Autodesk Inventor part; units mm, degrees
ref_plane "Work Plane1" through (0, 0, 10.47) normal (0, 0, 1) x (1, 0, 0)
ref_plane "YZ Plane" through (0, 0, 0) normal (1, 0, 0) x (0, 1, 0)
ref_plane "XZ Plane" through (0, 0, 0) normal (0, 1, 0) x (-1, 0, 0)
sketch "Base" plane through (0, 0, 0) normal (0, 0, 1) x (1, 0, 0)
  line L0 (-26.9, -20.25) -> (26.9, -20.25)
  line L1 (26.9, -20.25) -> (26.9, 20.25)
  line L2 (26.9, 20.25) -> (-26.9, 20.25)
  line L3 (-26.9, 20.25) -> (-26.9, -20.25)
  line L4 (-26.9, -20.25) -> (26.9, 20.25) construction
  line L5 (26.9, -20.25) -> (-26.9, 20.25) construction
  line L6 (-25.4, 16.25) -> (-22.9, 16.25) construction
  line L7 (-22.9, 16.25) -> (-22.9, 18.75) construction
  line L8 (-22.9, 18.75) -> (-25.4, 18.75) construction
  line L9 (-25.4, 18.75) -> (-25.4, 16.25) construction
  line L10 (-25.4, 16.25) -> (-22.9, 18.75) construction
  line L11 (-22.9, 16.25) -> (-25.4, 18.75) construction
  circle A0 centre (-24.15, 17.5) radius 1.25
  line L12 (-26.9, 0) -> (0, 0) construction
  line L13 (0, 20.25) -> (0, 0) construction
  circle A1 centre (-24.15, -17.5) radius 1.25
  circle A2 centre (24.15, 17.5) radius 1.25
  circle A3 centre (24.15, -17.5) radius 1.25
  point P0 (-25.4, 17.5)
  dimension "d0" = 53.8
  dimension "d1" = 40.5
  dimension "d2" = 1.5
  dimension "d3" = 1.5
  dimension "d4" = 2.5
extrude "BaseFeature" add sketch "Base" along normal blind 1.67
fillet "Fillet1" radius 2.5 4 edges at (-26.9, -20.25, 0.835) (26.9, -20.25, 0.835) (-26.9, 20.25, 0.835) (26.9, 20.25, 0.835)
sketch "Sketch2" plane through (0, 0, 1.67) normal (0, 0, 1) x (1, 0, 0)
  line L0 (-26.9, 17.75) -> (-26.9, -17.75)
  line L1 (-26.9, 0) -> (0, 0) construction
  line L2 (-26.4, 8.05) -> (-19.6, 8.05)
  line L3 (-19.6, 8.05) -> (-19.6, 1.25)
  line L4 (-19.6, 1.25) -> (-26.4, 1.25)
  line L5 (-26.4, 1.25) -> (-26.4, 8.05)
  line L6 (-26.4, -8.05) -> (-19.6, -8.05)
  line L7 (-19.6, -8.05) -> (-19.6, -1.25)
  line L8 (-19.6, -1.25) -> (-26.4, -1.25)
  line L9 (-26.4, -1.25) -> (-26.4, -8.05)
  dimension "d8" = 1.25
  dimension "d9" = 0.5
  dimension "d10" = 6.8
extrude "Extrusion2" add sketch "Sketch2" along normal blind 4.8
ref_plane "Work Plane1" through (0, 0, 10.47) normal (0, 0, 1) x (1, 0, 0)
sketch "Sketch3" plane through (0, 0, 10.47) normal (0, 0, 1) x (1, 0, 0)
  line L0 (-26.4, 8.05) -> (-19.6, 8.05)
  line L1 (-23, 8.05) -> (-23, 1.25) construction
  line L2 (-19.6, 1.25) -> (-26.4, 1.25)
  line L3 (-37.66, 0) -> (37.66, 0) construction
  line L4 (-26.4, 1.25) -> (-19.6, 1.25)
  line L5 (-19.6, 1.25) -> (-19.6, 8.05)
  line L6 (-19.6, 8.05) -> (-26.4, 8.05)
  line L7 (-26.4, 8.05) -> (-26.4, 1.25)
  line L8 (-25, 8.05) -> (-21, 8.05)
  line L9 (-21, 8.05) -> (-21, 1.25)
  line L10 (-21, 1.25) -> (-25, 1.25)
  line L11 (-25, 1.25) -> (-25, 8.05)
  point P0 (0, 0)
  dimension "d14" = 4
sketch "Sketch4" plane through (0, 0, 6.47) normal (0, 0, 1) x (1, 0, 0)
  line L0 (-26.4, 1.25) -> (-19.6, 1.25)
  line L1 (-19.6, 1.25) -> (-19.6, 8.05)
  line L2 (-19.6, 8.05) -> (-26.4, 8.05)
  line L3 (-26.4, 8.05) -> (-26.4, 1.25)
  point P0 (0, 0)
loft "Loft1" add profiles "Sketch3" section 2 edges at (-23, 1.25, 6.47) (-19.6, 4.65, 6.47) (-23, 8.05, 6.47) (-26.4, 4.65, 6.47) contours L0 L9 L2 L11
mirror "Mirror1" about plane through (0, 0, 0) normal (0, 1, 0) of "Loft1"
sketch "Sketch5" plane through (-25, 1.25, 10.47) normal (0, 0, 1) x (1, 0, 0)
  line L0 (0, 6.8) -> (0, 0)
  line L1 (0, 0) -> (4, 0)
  line L2 (4, 0) -> (4, 6.8)
  line L3 (4, 6.8) -> (0, 6.8)
  line L4 (-12.66, -1.25) -> (62.66, -1.25) construction
  line L5 (2, 6.8) -> (2, 0) construction
  circle A0 centre (2, 5.025) radius 1.5
  line L6 (0, 3.4) -> (4, 3.4) construction
  circle A1 centre (2, 1.775) radius 1.5
  point P0 (25, -1.25)
  dimension "d19" = 3
  dimension "d20" = 3.25
extrude "Extrusion3" cut sketch "Sketch5" against normal blind 3 contours A0 | A1
mirror "Mirror2" about plane through (0, 0, 0) normal (0, 1, 0) of "Extrusion3"
sketch "Sketch6" plane through (0, 0, 1.67) normal (0, 0, 1) x (1, 0, 0)
  line L0 (-24.4, -20.25) -> (24.4, -20.25)
  line L1 (-26.9, 17.75) -> (-26.9, -17.75)
  circle A0 centre (-14.4, -16.15) radius 4
  line L2 (-18.4, -16.15) -> (-18.4, -20.25) construction
  point P0 (0, 0)
  dimension "d23" = 8
  dimension "d24" = 4.1
  dimension "d25" = 8.5
extrude "Extrusion4" add sketch "Sketch6" along normal blind 12
fillet "Fillet2" radius 0.5 1 edges at (-18.4, -16.15, 13.67)
sketch "Sketch7" plane through (0, 0, 1.67) normal (0, 0, 1) x (1, 0, 0)
  line L0 (7.2, -9.65) -> (16.2, -9.65)
  line L1 (16.2, -9.65) -> (16.2, -23.65)
  line L2 (16.2, -23.65) -> (7.2, -23.65)
  line L3 (7.2, -23.65) -> (7.2, -9.65)
  line L4 (7.2, -23.65) -> (16.2, -23.65)
  line L5 (16.2, -23.65) -> (16.2, -20.25)
  line L6 (16.2, -20.25) -> (7.2, -20.25)
  line L7 (7.2, -20.25) -> (7.2, -23.65)
  line L8 (-24.4, -20.25) -> (24.4, -20.25)
  line L9 (26.9, -17.75) -> (26.9, 17.75)
  point P0 (0, 0)
  point P1 (11.7, -23.65)
  dimension "d29" = 9
  dimension "d30" = 14
  dimension "d31" = 3.4
  dimension "d32" = 10.7
extrude "Extrusion5" add sketch "Sketch7" along normal blind 10.7
sketch "Sketch8" plane through (7.2, -23.65, 1.67) normal (0, -1, 0) x (1, 0, 0)
  line L0 (0, 0) -> (9, 0)
  line L1 (9, 0) -> (9, 10.7)
  line L2 (0, 10.7) -> (9, 10.7)
  line L3 (0, 0) -> (0, 10.7)
  line L4 (4.5, 10.7) -> (4.5, 0) construction
  circle A0 centre (4.5, 6.2) radius 3.85
  point P0 (-7.2, -1.67)
  dimension "d35" = 7.7
  dimension "d36" = 4.5
extrude "Extrusion6" cut sketch "Sketch8" against normal blind 10.7 contours A0
sketch "Sketch9" plane through (0, 0, 1.67) normal (0, 0, 1) x (1, 0, 0)
  line L0 (11.77, 7.05) -> (29.4, 7.05)
  line L1 (29.4, 7.05) -> (29.4, 13.37)
  line L2 (29.4, 13.37) -> (11.77, 13.37)
  line L3 (11.77, 13.37) -> (11.77, 7.05)
  line L4 (24.4, 20.25) -> (-24.4, 20.25)
  line L5 (26.9, 13.37) -> (26.9, 7.05)
  line L6 (26.9, -17.75) -> (26.9, 17.75)
  point P0 (0, 0)
  dimension "d39" = 13.2
  dimension "d40" = 6.32
  dimension "d41" = 17.63
  dimension "d42" = 2.5
extrude "Extrusion7" add sketch "Sketch9" along normal blind 5 contours L3 L2 L5 L0
sketch "Sketch10" plane through (26.9, -17.75, 0) normal (1, 0, 0) x (0, 0, -1)
  line L0 (-1.67, 24.8) -> (-6.67, 24.8) construction
  line L1 (-1.67, 31.12) -> (-6.67, 31.12) construction
  line L2 (-6.67, 24.8) -> (-1.67, 31.12) construction
  circle A0 centre (-4.17, 27.96) radius 1.8
  point P0 (0, 17.75)
  dimension "d45" = 3.6
extrude "Extrusion8" cut sketch "Sketch10" against normal blind 5
sketch "Sketch11" plane through (26.9, -17.75, 0) normal (1, 0, 0) x (0, 0, -1)
  circle A0 centre (-4.17, 27.96) radius 1.8
  line L0 (-6.67, 24.8) -> (-6.67, 31.12)
  circle A1 centre (-4.17, 27.96) radius 2.5
  point P0 (0, 17.75)
extrude "Extrusion9" add sketch "Sketch11" along normal blind 2.5
sketch "Sketch12" plane through (0, 0, 0) normal (0, 0, -1) x (-1, 0, 0)
  line L0 (-26.9, 13.75) -> (-17.4, 13.75)
  line L1 (-17.4, 13.75) -> (-17.4, 4.25)
  line L2 (-17.4, 4.25) -> (-26.9, 4.25)
  line L3 (-26.9, 4.25) -> (-26.9, 13.75)
  line L4 (-26.9, -17.75) -> (-26.9, 17.75)
  line L5 (-24.4, 20.25) -> (24.4, 20.25)
  point P0 (0, 0)
  dimension "d50" = 9.5
  dimension "d51" = 6.5
extrude "Extrusion10" add sketch "Sketch12" along normal blind 5
sketch "Sketch13" plane through (0, 0, -5) normal (0, 0, -1) x (-1, 0, 0)
  line L0 (-17.4, 13.75) -> (-26.9, 13.75)
  line L1 (-26.9, 13.75) -> (-26.9, 4.25)
  line L2 (-26.9, 4.25) -> (-17.4, 4.25)
  line L3 (-17.4, 4.25) -> (-17.4, 13.75)
  circle A0 centre (-22.15, 9) radius 4
  line L4 (-17.4, 13.75) -> (-17.4, 4.25)
  line L5 (-26.9, 13.75) -> (-17.4, 4.25) construction
  point P0 (0, 0)
  dimension "d54" = 8
extrude "Extrusion11" add sketch "Sketch13" along normal blind 5 draft -4 contours A0
properties part number "FaceAudioBoard"
Here's how the part is built. I have some questions about the finished solid (model axes, mm). A direction names the side the tool comes from. Coordinates: 2 decimals unless noted, no trailing zeros. Order: outer loops, then holes, each group sorted by start corner. A loop starts at its lowest first (then second) coordinate and runs counter-clockwise, first axis right, second up. Notation, with made-up numbers: (71.25, -32.5) -> (78.25, -32.5) arc R21 cw to (78.25, -0.5) -> close; hole circle Ø6 at (-27.5, 21.5). An arc over 180 degrees is marked (long way). Return JSON: item names as keys, results as strings.
1) Thinking about a two-plate mould opening in X: for faces 5 (the cylindrical face through (26.187, 19.498, 0.847)), 6 (the flat face through (19, 13.37, 4)), 7 (the flat face through (7.2, -17, 7)), which applies, +X half, -X half, draft (parallel to the pull), parting line (faces both ways), or undercut?
Conclusion:
{"face 5": "+X half", "face 6": "draft", "face 7": "undercut"}
2) I'm going to push flat-ended pins straight in: P1, Ø1, axis at x = 19, z = 0, coming from the -Y side; P2, Ø5.5, axis at x = 24.5, z = -3.5, coming from the +Y side; P3, Ø6, axis at x = -9, y = 12, coming from the +Z side. Where does each tip first touch, or does it pass through?
Conclusion:
{"P1": "stops at y = -20.25", "P2": "stops at y = 13.75", "P3": "stops at z = 1.67"}
3) If we section it at A-A on z = 9.25: List the corners of the cut face in (x, y) for me (3 decimals).
Conclusion:
{"outline": "(-25.427, -8.05) -> (-20.573, -8.05) -> (-20.573, -1.25) -> (-25.427, -1.25) -> close; (-25.427, 1.25) -> (-20.573, 1.25) -> (-20.573, 8.05) -> (-25.427, 8.05) -> close; circle Ø8 at (-14.4, -16.15); (7.2, -23.65) -> (8.106, -23.65) -> (8.106, -12.95) -> (15.294, -12.95) -> (15.294, -23.65) -> (16.2, -23.65) -> (16.2, -9.65) -> (7.2, -9.65) -> close; hole circle Ø3 at (-23, -6.275); hole circle Ø3 at (-23, -3.025); hole circle Ø3 at (-23, 3.025); hole circle Ø3 at (-23, 6.275)"}
4) If we section it at C-C on x = -14.4: List the corners of the cut face in (y, z) for me.
Conclusion:
{"outline": "(-20.25, 0) -> (20.25, 0) -> (20.25, 1.67) -> (-12.15, 1.67) -> (-12.15, 13.17) arc R0.5 ccw to (-12.65, 13.67) -> (-19.65, 13.67) arc R0.5 ccw to (-20.15, 13.17) -> (-20.15, 1.67) -> (-20.25, 1.67) -> close"}
5) If I drill on probe 1 along Y at (x, z) = (24.15, 1); probe 2 along Y at (x, z) = (-23, 8.65) (3 decimals); probe 3 along X at (y, z) = (-16.5, 10.75), over which ranges is the centre line in solid material (lowest first)?
Conclusion:
{"probe 1": "y = -20.25 to -18.75, -16.25 to 16.25, 18.75 to 20.25", "probe 2": "y = -8.05 to -7.775, -4.775 to -4.525, -1.525 to -1.25, 1.25 to 1.525, 4.525 to 4.775, 7.775 to 8.05", "probe 3": "x = -18.38 to -10.42, 7.2 to 9.14, 14.26 to 16.2"}
6) If we section it at D-D on z = -3: List the corners of the cut face in (x, y) for me, plus the area to 4 significant figures.
Conclusion:
{"outline": "(17.4, 4.25) -> (26.9, 4.25) -> (26.9, 13.75) -> (17.4, 13.75) -> close", "area": "90.25 mm²"}
7) If we section it at B-B on y = -21: List the corners of the cut face in (x, z) for me, plus the area to 3 significant figures.
Conclusion:
{"outline": "(7.2, 1.67) -> (16.2, 1.67) -> (16.2, 12.37) -> (7.2, 12.37) -> close; hole circle Ø7.7 at (11.7, 7.87)", "area": "49.7 mm²"}
8) On a 3-axis mill with a long thin cutter (end or side, diameter ignored), from which of +Z, -Z, +X, -X, +Y, -Y can I reach the whole of each face in a straight line? I mean faces 1 (the flat face through (-23, 1.25, 6)), 2 (the cylindrical face through (-24.5, 3.1, 9)), 3 (the flat face through (-26.4, 5, 4)), 4 (the flat face through (16.2, -17, 7)). Say none if no direction works.
Conclusion:
{"face 1": "+Z, +X, -X", "face 2": "+Z", "face 3": "+Z, -X, +Y, -Y", "face 4": "+Z, +X, -Y"}
